Here's how the part is built. I have some questions about the finished solid (model axes, mm). Face numbers are marked on the shaded views. A direction names the side the tool comes from. Round coordinates to 2 decimals unless told otherwise and drop trailing zeros. Write each loop counter-clockwise with the first axis right and the second up, starting at its lowest first coordinate (ties: lowest second). Pieces come first, ordered by that corner, then holes. Notation, with made-up numbers: (33, 82) -> (58, 82) arc R13 cw to (58, 86) -> close; hole circle Ø7 at (61.5, -12). An arc over 180 degrees is marked (long way). Answer in a Markdown table with one row per item.
from build123d import *

# Parameters (mm, degrees)
F0_W     = 101.6
F0_H     = 101.6
F1_DEPTH = 5.08
F2_W     = 91.44
F2_H     = 5.08
F3_DEPTH = 101.6
F4_W     = 25.4
F4_H     = 50.8
F4_W_2   = 12.7
F4_H_2   = 12.7
F5_DEPTH = 5.08
F6_W     = 25.4
F6_H     = 25.4
F7_DEPTH = 5.08
F8_W     = 101.6
F8_H     = 101.6
F9_DEPTH = 5.08


with BuildPart() as f1:
    # F0 (on Top) → F1 (new body)
    with BuildSketch(Plane.XY):
        Rectangle(F0_W, F0_H)
    extrude(amount=F1_DEPTH)

    # F2 (on face) → F3 (join)
    with BuildSketch(Plane.XY.offset(5.08)):
        Polygon((-45.72, 50.8), (-50.8, 50.8), (-50.8, -50.8), (-45.72, -50.8), (-45.72, -45.72), (-45.72, 45.72), align=None)
        with Locations((0, 48.26)):
            Rectangle(F2_W, F2_H)
        Polygon((50.8, 50.8), (45.72, 50.8), (45.72, 45.72), (45.72, -45.72), (45.72, -50.8), (50.8, -50.8), align=None)
        with Locations((0, -48.26)):
            Rectangle(F2_W, F2_H)
    extrude(amount=F3_DEPTH)

    # F4 (on face) → F5 (cut, through all)
    with BuildSketch(Plane.XZ.offset(50.8)):
        with Locations((0, 30.48)):
            Rectangle(F4_W, F4_H)
        with Locations((-31.75, 93.98)):
            Rectangle(F4_W_2, F4_H_2)
        with Locations((31.75, 93.98)):
            Rectangle(F4_W_2, F4_H_2)
    extrude(amount=-F5_DEPTH, mode=Mode.SUBTRACT)

    # F6 (on face) → F7 (cut, through all)
    with BuildSketch(Plane(origin=(0, 50.8, 0), x_dir=(-1, 0, 0), z_dir=(0, 1, 0))):
        with Locations((-25.4, 81.28)):
            Rectangle(F6_W, F6_H)
        with Locations((25.4, 81.28)):
            Rectangle(F6_W, F6_H)
    extrude(amount=-F7_DEPTH, mode=Mode.SUBTRACT)

    # F8 (on face) → F9 (join)
    with BuildSketch(Plane.XY.offset(106.68)):
        Rectangle(F8_W, F8_H)
    extrude(amount=F9_DEPTH)


solid = f1.part
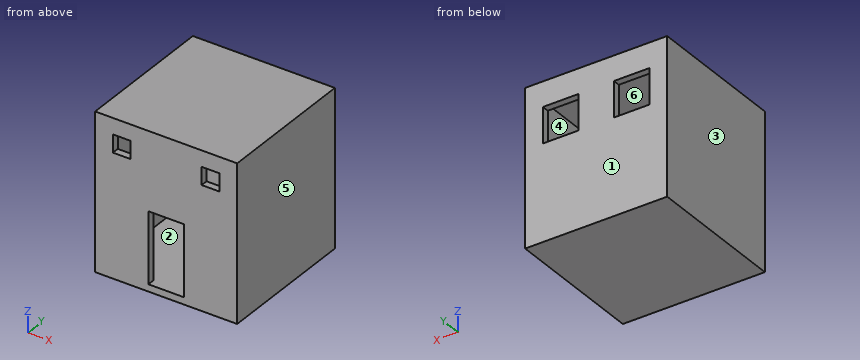
1) I want a section at A-A, the plane x = 35.5. List the corners of the cut face in (y, z) for me, and give its area (3 significant figures).
Response:
| item | result |
|---|---|
| outline | (-50.8, 0) -> (50.8, 0) -> (50.8, 68.58) -> (45.72, 68.58) -> (45.72, 5.08) -> (-45.72, 5.08) -> (-45.72, 87.63) -> (-50.8, 87.63) -> close; (-50.8, 100.33) -> (-45.72, 100.33) -> (-45.72, 106.68) -> (45.72, 106.68) -> (45.72, 93.98) -> (50.8, 93.98) -> (50.8, 111.76) -> (-50.8, 111.76) -> close |
| area | 1,870 mm^2 |
2) I need wall thicknesses on line 1 (Z direction, x = 9, y = 32.5); line 2 (X direction, y = 15, z = 57.5). Which ranges of each line are inside material? Lowest first, please. Write a range as [from, to].
Response:
| item | result |
|---|---|
| line 1 | z = [0, 5.08], [106.68, 111.76] |
| line 2 | x = [-50.8, -45.72], [45.72, 50.8] |
3) I want a section at D-D, the plane x = -5. List the corners of the cut face in (y, z) for me, and give its area (3 significant figures).
Response:
| item | result |
|---|---|
| outline | (-50.8, 0) -> (50.8, 0) -> (50.8, 111.76) -> (-50.8, 111.76) -> (-50.8, 55.88) -> (-45.72, 55.88) -> (-45.72, 106.68) -> (45.72, 106.68) -> (45.72, 5.08) -> (-50.8, 5.08) -> close |
| area | 1,810 mm^2 |
4) I want a section at B-B, the plane z = 79.5. List the corners of the cut face in (x, y) for me.
Response:
| item | result |
|---|---|
| outline | (-50.8, -50.8) -> (50.8, -50.8) -> (50.8, 50.8) -> (38.1, 50.8) -> (38.1, 45.72) -> (45.72, 45.72) -> (45.72, -45.72) -> (-45.72, -45.72) -> (-45.72, 45.72) -> (-38.1, 45.72) -> (-38.1, 50.8) -> (-50.8, 50.8) -> close; (-12.7, 45.72) -> (12.7, 45.72) -> (12.7, 50.8) -> (-12.7, 50.8) -> close |
5) I want a section at C-C, the plane y = -17. List the corners of the cut face in (x, z) for me, and give its area (3 significant figures).
Response:
| item | result |
|---|---|
| outline | (-50.8, 0) -> (50.8, 0) -> (50.8, 111.76) -> (-50.8, 111.76) -> close; hole (-45.72, 5.08) -> (45.72, 5.08) -> (45.72, 106.68) -> (-45.72, 106.68) -> close |
| area | 2,060 mm^2 |
6) Which directions (+Z, -Z, +X, -X, +Y, -Y) give clear straight access to the entire face, cutting with the end or side of a thin tool? Please do the marked faces 1 and 2.
Response:
| item | result |
|---|---|
| face 1 | +Z, -Z, +X, -X, +Y |
| face 2 | none |
7) We'd pull the mould along X, two halves only. Please class the marked faces 3, 4, 5 and 6: +X half, -X half, draft (parallel to the pull), parting line (faces both ways), or undercut.
Response:
| item | result |
|---|---|
| face 3 | -X half |
| face 4 | undercut |
| face 5 | +X half |
| face 6 | undercut |
